from build123d import *
from OCP.BRepFilletAPI import BRepFilletAPI_MakeChamfer

# Parameters (mm, degrees)
SKETCH1_W           = 150
SKETCH1_H           = 150
BOSS_EXTRUDE1_DEPTH = 1
SKETCH2_W           = 150
SKETCH2_H           = 150
BOSS_EXTRUDE2_DEPTH = 60
CHAMFER1_SIZE       = 60
CHAMFER1_SIZE2      = 34.641016151
CHAMFER2_SIZE       = 5
CHAMFER2_SIZE2      = 2.886751346
CHAMFER3_SIZE       = 1
CHAMFER3_SIZE2      = 0.577350269
CHAMFER4_SIZE       = 1
CHAMFER4_SIZE2      = 0.577350269
SKETCH3_W           = 145
SKETCH3_H           = 145
BOSS_EXTRUDE3_DEPTH = 4.5


with BuildPart() as part:
    # Sketch1 → Boss-Extrude1 (new body)
    with BuildSketch(Plane(origin=(0, 0, 0), x_dir=(1, 0, 0), z_dir=(0, 1, 0))):
        Rectangle(SKETCH1_W, SKETCH1_H)
    extrude(amount=BOSS_EXTRUDE1_DEPTH)

    # Sketch2 → Boss-Extrude2 (add)
    with BuildSketch(Plane(origin=(0, 1, 0), x_dir=(1, 0, 0), z_dir=(0, 1, 0))):
        Rectangle(SKETCH2_W, SKETCH2_H)
    extrude(amount=BOSS_EXTRUDE2_DEPTH)

    # Chamfer1: one chamfer whose edges measure the first distance from different faces: ONE call of the kernel's chamfer builder (chamfer() names one face for all edges)
    chamfer1_edges_1 = [part.edges().sort_by_distance(p)[0] for p in [
        (75, 61, 0),
    ]]
    chamfer1_side_1 = [part.faces().sort_by_distance(p)[0] for p in [
        (75, 30.5, 0),
    ]]
    chamfer1_edges_2 = [part.edges().sort_by_distance(p)[0] for p in [
        (-75, 61, 0),
    ]]
    chamfer1_side_2 = [part.faces().sort_by_distance(p)[0] for p in [
        (-75, 30.5, 0),
    ]]
    chamfer1 = BRepFilletAPI_MakeChamfer(part.part.solid().wrapped)
    for e in chamfer1_edges_1:
        chamfer1.Add(CHAMFER1_SIZE, CHAMFER1_SIZE2, e.wrapped, chamfer1_side_1[0].wrapped)  # the first distance lies on this face
    for e in chamfer1_edges_2:
        chamfer1.Add(CHAMFER1_SIZE, CHAMFER1_SIZE2, e.wrapped, chamfer1_side_2[0].wrapped)  # the first distance lies on this face
    add(Compound.cast(chamfer1.Shape()), mode=Mode.REPLACE)

    # Chamfer2: one chamfer whose edges measure the first distance from different faces: ONE call of the kernel's chamfer builder (chamfer() names one face for all edges)
    chamfer2_edges_1 = [part.edges().sort_by_distance(p)[0] for p in [
        (0, 61, -75),
    ]]
    chamfer2_side_1 = [part.faces().sort_by_distance(p)[0] for p in [
        (0, 27.413848587, -75),
    ]]
    chamfer2_edges_2 = [part.edges().sort_by_distance(p)[0] for p in [
        (0, 61, 75),
    ]]
    chamfer2_side_2 = [part.faces().sort_by_distance(p)[0] for p in [
        (0, 27.413848587, 75),
    ]]
    chamfer2 = BRepFilletAPI_MakeChamfer(part.part.solid().wrapped)
    for e in chamfer2_edges_1:
        chamfer2.Add(CHAMFER2_SIZE, CHAMFER2_SIZE2, e.wrapped, chamfer2_side_1[0].wrapped)  # the first distance lies on this face
    for e in chamfer2_edges_2:
        chamfer2.Add(CHAMFER2_SIZE, CHAMFER2_SIZE2, e.wrapped, chamfer2_side_2[0].wrapped)  # the first distance lies on this face
    add(Compound.cast(chamfer2.Shape()), mode=Mode.REPLACE)

    # Chamfer3: one chamfer whose edges measure the first distance from different faces: ONE call of the kernel's chamfer builder (chamfer() names one face for all edges)
    chamfer3_edges_1 = [part.edges().sort_by_distance(p)[0] for p in [
        (-75, 0.5, -75),
    ]]
    chamfer3_side_1 = [part.faces().sort_by_distance(p)[0] for p in [
        (0, 25.462591876, -75),
    ]]
    chamfer3_edges_2 = [part.edges().sort_by_distance(p)[0] for p in [
        (75, 0.5, -75),
    ]]
    chamfer3_side_2 = [part.faces().sort_by_distance(p)[0] for p in [
        (75, 0.5, 0),
    ]]
    chamfer3_edges_3 = [part.edges().sort_by_distance(p)[0] for p in [
        (75, 0.5, 75),
    ]]
    chamfer3_side_3 = [part.faces().sort_by_distance(p)[0] for p in [
        (0, 25.462591876, 75),
    ]]
    chamfer3_edges_4 = [part.edges().sort_by_distance(p)[0] for p in [
        (-75, 0.5, 75),
    ]]
    chamfer3_side_4 = [part.faces().sort_by_distance(p)[0] for p in [
        (-75, 0.5, 0),
    ]]
    chamfer3 = BRepFilletAPI_MakeChamfer(part.part.solid().wrapped)
    for e in chamfer3_edges_1:
        chamfer3.Add(CHAMFER3_SIZE, CHAMFER3_SIZE2, e.wrapped, chamfer3_side_1[0].wrapped)  # the first distance lies on this face
    for e in chamfer3_edges_2:
        chamfer3.Add(CHAMFER3_SIZE, CHAMFER3_SIZE2, e.wrapped, chamfer3_side_2[0].wrapped)  # the first distance lies on this face
    for e in chamfer3_edges_3:
        chamfer3.Add(CHAMFER3_SIZE, CHAMFER3_SIZE2, e.wrapped, chamfer3_side_3[0].wrapped)  # the first distance lies on this face
    for e in chamfer3_edges_4:
        chamfer3.Add(CHAMFER3_SIZE, CHAMFER3_SIZE2, e.wrapped, chamfer3_side_4[0].wrapped)  # the first distance lies on this face
    add(Compound.cast(chamfer3.Shape()), mode=Mode.REPLACE)

    # Chamfer4: one chamfer whose edges measure the first distance from different faces: ONE call of the kernel's chamfer builder (chamfer() names one face for all edges)
    chamfer4_edges_1 = [part.edges().sort_by_distance(p)[0] for p in [
        (-58.622867597, 29.366025404, -75),
        (-58.834192463, 29, 75),
    ]]
    chamfer4_side_1 = [part.faces().sort_by_distance(p)[0] for p in [
        (-57.703873012, 30.957770718, 7.84e-06),
    ]]
    chamfer4_edges_2 = [part.edges().sort_by_distance(p)[0] for p in [
        (58.834192463, 29, -75),
        (58.622867597, 29.366025404, 75),
    ]]
    chamfer4_side_2 = [part.faces().sort_by_distance(p)[0] for p in [
        (57.703873012, 30.957770718, -7.84e-06),
    ]]
    chamfer4 = BRepFilletAPI_MakeChamfer(part.part.solid().wrapped)
    for e in chamfer4_edges_1:
        chamfer4.Add(CHAMFER4_SIZE, CHAMFER4_SIZE2, e.wrapped, chamfer4_side_1[0].wrapped)  # the first distance lies on this face
    for e in chamfer4_edges_2:
        chamfer4.Add(CHAMFER4_SIZE, CHAMFER4_SIZE2, e.wrapped, chamfer4_side_2[0].wrapped)  # the first distance lies on this face
    add(Compound.cast(chamfer4.Shape()), mode=Mode.REPLACE)

    # Sketch3 → Boss-Extrude3 (add)
    with BuildSketch(Plane(origin=(0, 0, 0), x_dir=(-1, 0, 0), z_dir=(0, -1, 0))):
        Rectangle(SKETCH3_W, SKETCH3_H)
    extrude(amount=BOSS_EXTRUDE3_DEPTH)


solid = part.part
Check sheet for the modelled part. Datum: model origin and axes. Units: mm. A direction names the side the tool comes from. Give positions to 0.01 mm unless a question says otherwise; leave off trailing zeros. Loops run counter-clockwise (first coordinate to the right, second up) from the corner with the lowest first, then second, coordinate; pieces in that order, holes last. Notation, with made-up numbers: M 13.25,18.25 L 33.25,18.25 A16 cw 33.25,41.25 Z; hole C 11,-16.75 d11. An arc over 180 degrees is marked long. Return JSON: item names as keys, results as strings. Group by question number.
1. Cross-section at C-C on x = -48.5. Record the boundary of the cut face in (y, z), plus the area to 3 significant figures.
2. Cross-section at D-D on y = 43. Record the boundary of the cut face in (x, z).
3. Go/stop test with flat-tipped pins: pin 1 (3.5 mm diameter, centred on y = -2.5, z = 32.5, fed in from +X); pin 2 (5 mm diameter, centred on y = 40.5, z = 45.5, fed in from -X); pin 3 (10 mm diameter, centred on y = 50.5, z = -11.5, fed in from +X). Record where each tip stops, or that it passes through.
4. Cross-section at B-B on y = 51.5. Record the boundary of the cut face in (x, z).
5. Cross-section at A-A on z = 6. Record the boundary of the cut face in (x, y).
6. Thickness scan on L1, parallel to X at y = 6, z = 50; L2, parallel to X at y = -1.5, z = -54; L3, parallel to Y at x = -48.5, z = -40.5. Record the ranges inside material, lowest first.
7. Tool access check on faces 1 (the flat face through (1, -2, -72.5)), 2 (the flat face through (1, -2, 72.5)), 3 (the flat face through (72.5, -2, 1)), 4 (the flat face through (-72.5, -2, 1)). Record the directions out of +Z, -Z, +X, -X, +Y, -Y that give a thin tool (end or side, any length) a straight path to the whole face; none if there is none.
Return value:
{
 "1": {"outline": "M -4.5,-72.5 L 0,-72.5 L 0,-75 L 45.74,-75 L 46.9,-74 L 46.9,74 L 45.74,75 L 0,75 L 0,72.5 L -4.5,72.5 Z", "area": "7,690 mm^2"},
 "2": {"outline": "M -50.75,-74 L -50.08,-75 L 50.08,-75 L 50.75,-74 L 50.75,74 L 50.08,75 L -50.08,75 L -50.75,74 Z"},
 "3": {"pin 1": "x = 72.5", "pin 2": "x = -53.64", "pin 3": "x = 49.31"},
 "4": {"outline": "M -45.84,-74 L -45.18,-75 L 45.18,-75 L 45.84,-74 L 45.84,74 L 45.18,75 L -45.18,75 L -45.84,74 Z"},
 "5": {"outline": "M -75,0 L -72.5,0 L -72.5,-4.5 L 72.5,-4.5 L 72.5,0 L 75,0 L 75,1 L 40.36,61 L -40.36,61 L -75,1 Z"},
 "6": {"L1": "-72.11 to 72.11", "L2": "-72.5 to 72.5", "L3": "-4.5 to 46.9"},
 "7": {"face 1": "-Z, +X, -X, -Y", "face 2": "+Z, +X, -X, -Y", "face 3": "+Z, -Z, +X, -Y", "face 4": "+Z, -Z, -X, -Y"}
}
